Input: dimensioned drawing with shaded views. Units: mm. Origin: part minimum x, y, z. Give positions to 0.01 mm unless a question says otherwise; leave off trailing zeros. Loops run counter-clockwise (first coordinate to the right, second up) from the corner with the lowest first, then second, coordinate; pieces in that order, holes last. Notation, with made-up numbers: (-16.5, 65) -> (38.5, 65) arc R23 ccw to (38.5, 91) -> close; hole circle Ø2 at (-10, -21). An arc over 180 degrees is marked (long way). Answer as a JSON object with one key per item and string values.
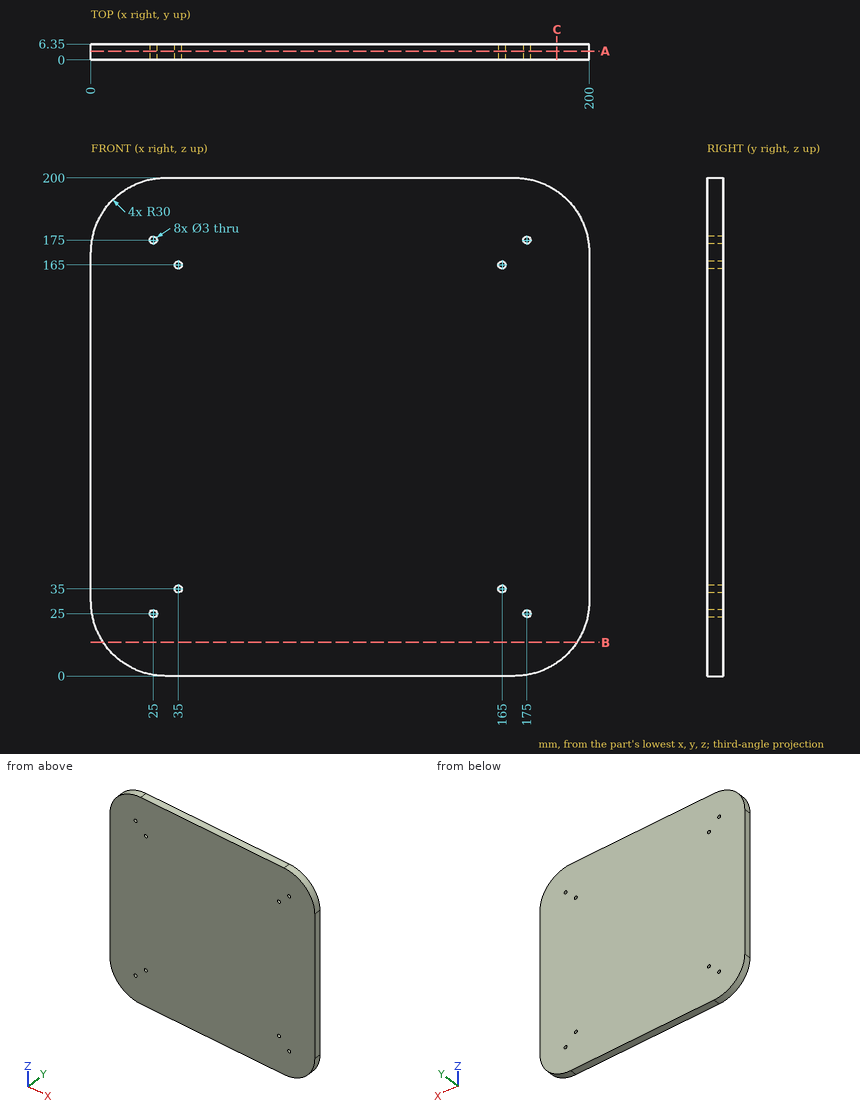
Q1. Section A-A, the plane y = 3.5. Give the number of separate pieces and of enclosed holes in the cut face, then the cut area to 3 significant figures.
Evaluation:
{"separate pieces": "1", "enclosed holes": "8", "area": "39,200 mm2"}
Q2. Ray query, line 1 along Z through (x, y) = (35, 4.25); line 2 along Z through (x, y) = (175, 4.5). Return the intervals inside material, ascending.
Evaluation:
{"line 1": "z = 0 to 33.5, 36.5 to 163.5, 166.5 to 200", "line 2": "z = 0.42 to 23.5, 26.5 to 173.5, 176.5 to 199.58"}
Q3. Section B-B, the plane z = 13.5. Return the cut outline in (x, y), then the cut area to 3 significant figures.
Evaluation:
{"outline": "(4.95, 0) -> (195.05, 0) -> (195.05, 6.35) -> (4.95, 6.35) -> close", "area": "1,210 mm2"}
Q4. Section C-C, the plane x = 187. Return the cut outline in (y, z), then the cut area to 3 significant figures.
Evaluation:
{"outline": "(0, 5.28) -> (6.35, 5.28) -> (6.35, 194.72) -> (0, 194.72) -> close", "area": "1,200 mm2"}
